Work out the finished part from the listing and answer in its coordinate system (mm). Face numbers are marked on the shaded views. A direction names the side the tool comes from. Round coordinates to 2 decimals unless told otherwise and drop trailing zeros. Order: outer loops, then holes, each group sorted by start corner. A loop starts at its lowest first (then second) coordinate and runs counter-clockwise, first axis right, second up. Notation, with made-up numbers: (29.5, 18.5) - (73.5, 18.5) arc R35 ccw to (73.5, 52.5) - close; hole circle Ø2 at (2.5, 65). An arc over 180 degrees is marked (long way). Put each result on its own line as item: value.
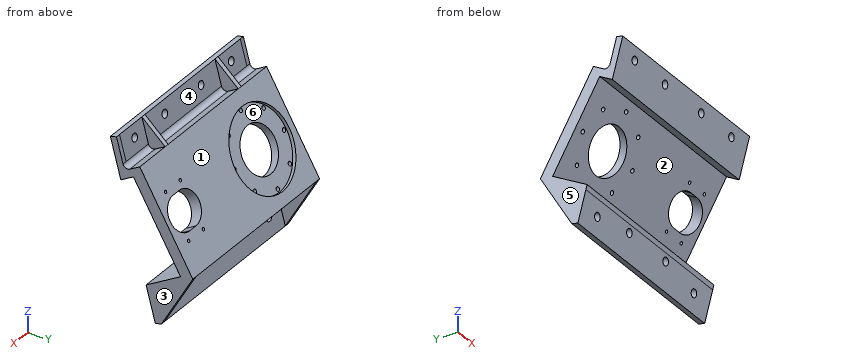
```python
from build123d import *

# Parameters (mm, degrees)
EXTRUDE_1_DEPTH      = 30
SKETCH_2_R           = 44.45
CUT_EXTRUDE_1_DEPTH  = 4
SKETCH_3_R           = 25.5
SKETCH_3_R_2         = 2.25
CUT_EXTRUDE_2_DEPTH  = 188.619295383
CUT_EXTRUDE_3_DEPTH  = 189.215302247
SKETCH_5_R           = 1.65
CUT_EXTRUDE_4_DEPTH  = 189.215302247
EXTRUDE_START        = -30
EXTRUDE_2_DEPTH      = 30
CUT_EXTRUDE_5_DEPTH  = 198.040604952
CUT_EXTRUDE_7_DEPTH  = 233.432785983
CUT_EXTRUDE_8_DEPTH  = 233.432785983
CUT_EXTRUDE_9_DEPTH  = 233.432785983
FILLET_1_R           = 5
CUT_EXTRUDE_10_DEPTH = 233.432785983
EXTRUDE_START_2      = -5
EXTRUDE_3_DEPTH      = 5
EXTRUDE_4_DEPTH      = 5
SKETCH_14_R          = 4.25
CUT_EXTRUDE_11_DEPTH = 189.364728478
SKETCH_16_W          = 43
SKETCH_16_H          = 30
CUT_EXTRUDE_12_DEPTH = 233.432785983
EXTRUDE_7_REACH      = 188.592
SKETCH_18_W          = 210
SKETCH_18_H          = 5
EXTRUDE_8_DEPTH      = 210
EXTRUDE_9_DEPTH      = 5
EXTRUDE_10_DEPTH     = 5
SKETCH_22_R          = 4.25
CUT_EXTRUDE_13_DEPTH = 187.984035343
FILLET_2_R           = 5
EXTRUDE_11_DEPTH     = 2.5
CUT_EXTRUDE_START    = -5
CUT_EXTRUDE_16_DEPTH = 5
EXTRUDE_12_DEPTH     = 2.5
CUT_EXTRUDE_18_DEPTH = 5
CUT_EXTRUDE_19_DEPTH = 366.180703078


with BuildPart() as part:
    # 草图1 → 凸台-拉伸1 (new body)
    with BuildSketch(Plane(origin=(0, 0, 0), x_dir=(1, 0, 0), z_dir=(0, 1, 0))):
        with BuildLine():
            Line((170, 31.93), (170, -31.93))
            ThreePointArc((170, -31.93), (167.781993847, -38.210172909), (162.111885646, -41.704453387))
            Line((162.111885646, -41.704453387), (15.839142344, -73.308400404))
            ThreePointArc((15.839142344, -73.308400404), (-75, 0), (15.839142344, 73.308400404))
            Line((15.839142344, 73.308400404), (162.111885646, 41.704453387))
            ThreePointArc((162.111885646, 41.704453387), (167.781993847, 38.210172909), (170, 31.93))
        make_face()
    extrude(amount=EXTRUDE_1_DEPTH)

    # 草图2 → 切除-拉伸1 (cut)
    with BuildSketch(Plane(origin=(0, 30, 0), x_dir=(1, 0, 0), z_dir=(0, 1, 0))):
        with Locations(Location((0, 0, 0), (0, 0, 270))):
            Circle(SKETCH_2_R)
    extrude(amount=-CUT_EXTRUDE_1_DEPTH, mode=Mode.SUBTRACT)

    # 草图3 → 切除-拉伸2 (cut, through all)
    with BuildSketch(Plane(origin=(0, 26, 0), x_dir=(1, 0, 0), z_dir=(0, 1, 0))):
        with Locations(Location((0, 0, 0), (0, 0, 270))):
            Circle(SKETCH_3_R)
        with Locations(Location((0, 41, 0), (0, 0, 270))):
            Circle(SKETCH_3_R_2)
        with Locations(Location((28.991378029, 28.991378029, 0), (0, 0, 270))):
            Circle(SKETCH_3_R_2)
        with Locations(Location((41, 0, 0), (0, 0, 270))):
            Circle(SKETCH_3_R_2)
        with Locations(Location((28.991378029, -28.991378029, 0), (0, 0, 270))):
            Circle(SKETCH_3_R_2)
        with Locations(Location((0, -41, 0), (0, 0, 270))):
            Circle(SKETCH_3_R_2)
        with Locations(Location((-28.991378029, -28.991378029, 0), (0, 0, 270))):
            Circle(SKETCH_3_R_2)
        with Locations(Location((-41, 0, 0), (0, 0, 270))):
            Circle(SKETCH_3_R_2)
        with Locations(Location((-28.991378029, 28.991378029, 0), (0, 0, 270))):
            Circle(SKETCH_3_R_2)
    extrude(amount=-CUT_EXTRUDE_2_DEPTH, mode=Mode.SUBTRACT)

    # 草图4 → 切除-拉伸3 (cut, through all)
    with BuildSketch(Plane(origin=(0, 30, 0), x_dir=(1, 0, 0), z_dir=(0, 1, 0))):
        with BuildLine():
            Line((124, 18.5), (134, 18.5))
            ThreePointArc((134, 18.5), (152.5, 0), (134, -18.5))
            Line((134, -18.5), (124, -18.5))
            ThreePointArc((124, -18.5), (105.5, 0), (124, 18.5))
        make_face()
    extrude(amount=-CUT_EXTRUDE_3_DEPTH, mode=Mode.SUBTRACT)

    # 草图5 → 切除-拉伸4 (cut, through all)
    with BuildSketch(Plane(origin=(0, 30, 0), x_dir=(1, 0, 0), z_dir=(0, 1, 0))):
        with Locations(Location((116.75, 25.5, 0), (0, 0, 270))):
            Circle(SKETCH_5_R)
        with Locations(Location((141.25, 25.5, 0), (0, 0, 270))):
            Circle(SKETCH_5_R)
        with Locations(Location((141.25, -25.5, 0), (0, 0, 270))):
            Circle(SKETCH_5_R)
        with Locations(Location((116.75, -25.5, 0), (0, 0, 270))):
            Circle(SKETCH_5_R)
    extrude(amount=-CUT_EXTRUDE_4_DEPTH, mode=Mode.SUBTRACT)

    # 草图6 → 凸台-拉伸2 (add)
    with BuildSketch(Plane(origin=(0, 30, 0), x_dir=(1, 0, 0), z_dir=(0, 1, 0)).offset(EXTRUDE_START)):
        with BuildLine():
            Line((158, 95), (-52, 95))
            Line((-52, 95), (-52, 54.046276467))
            ThreePointArc((-52, 54.046276467), (-20.48558667, 72.148047366), (15.839142344, 73.308400404))
            Line((15.839142344, 73.308400404), (158, 42.592874655))
            Line((158, 42.592874655), (158, 95))
        make_face()
        with BuildLine():
            ThreePointArc((15.839142344, -73.308400404), (-20.48558667, -72.148047366), (-52, -54.046276467))
            Line((-52, -54.046276467), (-52, -95))
            Line((-52, -95), (158, -95))
            Line((158, -95), (158, -42.592874655))
            Line((158, -42.592874655), (15.839142344, -73.308400404))
        make_face()
    extrude(amount=EXTRUDE_2_DEPTH)

    # 草图7 → 切除-拉伸5 (cut, through all)
    with BuildSketch(Plane(origin=(0, 30, 0), x_dir=(1, 0, 0), z_dir=(0, 1, 0))):
        with BuildLine():
            Line((-52, 54.046276467), (-52, -54.046276467))
            ThreePointArc((-52, -54.046276467), (-75, 0), (-52, 54.046276467))
        make_face()
        with BuildLine():
            Line((158, 42.592874655), (158, -42.592874655))
            Line((158, -42.592874655), (162.111885646, -41.704453387))
            ThreePointArc((162.111885646, -41.704453387), (167.781993847, -38.210172909), (170, -31.93))
            Line((170, -31.93), (170, 31.93))
            ThreePointArc((170, 31.93), (167.781993847, 38.210172909), (162.111885646, 41.704453387))
            Line((162.111885646, 41.704453387), (158, 42.592874655))
        make_face()
    extrude(amount=-CUT_EXTRUDE_5_DEPTH, mode=Mode.SUBTRACT)

    # 草图9 → 切除-拉伸7 (cut, through all)
    with BuildSketch(Plane.ZY.offset(52)):
        Polygon((-95, 20), (-60, 10.621778265), (-60, 30), (-95, 30), align=None)
    extrude(amount=-CUT_EXTRUDE_7_DEPTH, mode=Mode.SUBTRACT)

    # 草图10 → 切除-拉伸8 (cut, through all)
    with BuildSketch(Plane.ZY.offset(52)):
        Polygon((-95, 12.753066737), (-52, 1.231251463), (-52, 0), (-95, 0), align=None)
    extrude(amount=-CUT_EXTRUDE_8_DEPTH, mode=Mode.SUBTRACT)

    # 草图8 → 切除-拉伸9 (cut, through all)
    with BuildSketch(Plane.ZY.offset(52)):
        Polygon((0, 0), (52, 0), (52, 17.3), (-52, 17.3), (-52, 0), align=None)
    extrude(amount=-CUT_EXTRUDE_9_DEPTH, mode=Mode.SUBTRACT)

    # 圆角1
    fillet_1_edges = [part.edges().sort_by_distance(p)[0] for p in [
        (53, 10.621778265, -60),
    ]]
    fillet(fillet_1_edges, radius=FILLET_1_R)

    # 草图11 → 切除-拉伸10 (cut, through all)
    with BuildSketch(Plane.ZY.offset(52)):
        Polygon((-95, 12.753066737), (-93.188266684, 19.514547521), (-95, 20), align=None)
    extrude(amount=-CUT_EXTRUDE_10_DEPTH, mode=Mode.SUBTRACT)

    # 草图12 → 凸台-拉伸3 (add)
    with BuildSketch(Plane.ZY.offset(52).offset(EXTRUDE_START_2)):
        with BuildLine():
            Line((-93.188266684, 19.514547521), (-60, 30))
            Line((-60, 30), (-60, 17.137905129))
            ThreePointArc((-60, 17.137905129), (-61.956192855, 13.171138428), (-66.294095226, 12.308275998))
            Line((-66.294095226, 12.308275998), (-93.188266684, 19.514547521))
        make_face()
    extrude(amount=EXTRUDE_3_DEPTH)

    # 草图13 → 凸台-拉伸4 (add)
    with BuildSketch(Plane(origin=(158, 0, 0), x_dir=(0, 0, -1), z_dir=(1, 0, 0))):
        with BuildLine():
            Line((66.294095226, 12.308275998), (93.188266684, 19.514547521))
            Line((93.188266684, 19.514547521), (60, 30))
            Line((60, 30), (60, 17.137905129))
            ThreePointArc((60, 17.137905129), (61.956192855, 13.171138428), (66.294095226, 12.308275998))
        make_face()
    extrude(amount=-EXTRUDE_4_DEPTH)

    # 草图14 → 切除-拉伸11 (cut, through all)
    with BuildSketch(Plane(origin=(0, -5.089745962, -1.36379332), x_dir=(1, 0, 0), z_dir=(0, 0.9659258262890681, 0.2588190451025214))):
        with Locations(Location((-27, 82.063690052, 0), (0, 0, 270))):
            Circle(SKETCH_14_R)
        with Locations(Location((23, 82.063690052, 0), (0, 0, 270))):
            Circle(SKETCH_14_R)
        with Locations(Location((83, 82.063690052, 0), (0, 0, 270))):
            Circle(SKETCH_14_R)
        with Locations(Location((133, 82.063690052, 0), (0, 0, 270))):
            Circle(SKETCH_14_R)
    extrude(amount=-CUT_EXTRUDE_11_DEPTH, mode=Mode.SUBTRACT)

    # 草图16 → 切除-拉伸12 (cut, through all)
    with BuildSketch(Plane.ZY.offset(52)):
        with Locations((73.5, 15)):
            Rectangle(SKETCH_16_W, SKETCH_16_H)
    extrude(amount=-CUT_EXTRUDE_12_DEPTH, mode=Mode.SUBTRACT)

    # 凸台-拉伸7: up to this plane
    extrude_7_end = Plane(origin=(0, -11.851226746, -3.175526636), z_dir=(0, -0.9659258262890681, -0.25881904510252146))
    # 草图18 → 凸台-拉伸7 (add, up to the surface)
    with BuildSketch(Plane(origin=(0, 30, 0), x_dir=(1, 0, 0), z_dir=(0, 1, 0)), mode=Mode.PRIVATE) as extrude_7_sk1:
        with Locations((53, -54.5)):
            Rectangle(SKETCH_18_W, SKETCH_18_H)
    extrude_7_tool1 = split(extrude(extrude_7_sk1.sketch, amount=-EXTRUDE_7_REACH, mode=Mode.PRIVATE), bisect_by=extrude_7_end, keep=Keep.BOTH, mode=Mode.PRIVATE)
    add(extrude_7_tool1.solids().sort_by_distance((53, 30, 54.5))[0])

    # 草图19 → 凸台-拉伸8 (add)
    with BuildSketch(Plane.ZY.offset(52)):
        Polygon((57, -27.975210512), (90.188266684, -36.867979769), (92, -30.106498985), (57, -20.72827725), align=None)
    extrude(amount=-EXTRUDE_8_DEPTH)

    # 草图20 → 凸台-拉伸9 (add)
    with BuildSketch(Plane.ZY.offset(52)):
        Polygon((92, -30.106498985), (57, -20.72827725), (57, 30), align=None)
    extrude(amount=-EXTRUDE_9_DEPTH)

    # 草图21 → 凸台-拉伸10 (add)
    with BuildSketch(Plane(origin=(158, 0, 0), x_dir=(0, 0, -1), z_dir=(1, 0, 0))):
        Polygon((-57, 30), (-92, -30.106498985), (-57, -20.72827725), align=None)
    extrude(amount=-EXTRUDE_10_DEPTH)

    # 草图22 → 切除-拉伸13 (cut, through all)
    with BuildSketch(Plane(origin=(0, -5.089745962, -1.36379332), x_dir=(1, 0, 0), z_dir=(0, 0.9659258262890686, 0.25881904510251946))):
        with Locations(Location((-27, -77.936309948, 0), (0, 0, 270))):
            Circle(SKETCH_22_R)
        with Locations(Location((23, -69.936309948, 0), (0, 0, 270))):
            Circle(SKETCH_22_R)
        with Locations(Location((83, -69.936309948, 0), (0, 0, 270))):
            Circle(SKETCH_22_R)
        with Locations(Location((133, -77.936309948, 0), (0, 0, 270))):
            Circle(SKETCH_22_R)
    extrude(amount=-CUT_EXTRUDE_13_DEPTH, mode=Mode.SUBTRACT)

    # 圆角2
    fillet_2_edges = [part.edges().sort_by_distance(p)[0] for p in [
        (53, -20.72827725, 57),
    ]]
    fillet(fillet_2_edges, radius=FILLET_2_R)

    # 草图27 → 凸台-拉伸11 (add, symmetric)
    with BuildSketch(Plane(origin=(113.5, 0, 0), x_dir=(0, 0, -1), z_dir=(1, 0, 0))):
        with BuildLine():
            Line((60, 30), (60, 17.137905129))
            ThreePointArc((60, 17.137905129), (61.956192855, 13.171138428), (66.294095226, 12.308275998))
            Line((66.294095226, 12.308275998), (93.188266684, 19.514547521))
            Line((93.188266684, 19.514547521), (60, 30))
        make_face()
    extrude(amount=EXTRUDE_11_DEPTH, both=True)

    # 草图29 → 切除-拉伸16 (cut)
    with BuildSketch(Plane.ZY.offset(-153).offset(CUT_EXTRUDE_START)):
        with BuildLine():
            Line((-60, 17.137905129), (-60, 30))
            Line((-60, 30), (-93.188266684, 19.514547521))
            Line((-93.188266684, 19.514547521), (-66.294095226, 12.308275998))
            ThreePointArc((-66.294095226, 12.308275998), (-61.956192855, 13.171138428), (-60, 17.137905129))
        make_face()
    extrude(amount=CUT_EXTRUDE_16_DEPTH, mode=Mode.SUBTRACT)

    # 草图30 → 凸台-拉伸12 (add, symmetric)
    with BuildSketch(Plane.ZY.offset(7.5)):
        with BuildLine():
            Line((-93.188266684, 19.514547521), (-66.294095226, 12.308275998))
            ThreePointArc((-66.294095226, 12.308275998), (-61.956192855, 13.171138428), (-60, 17.137905129))
            Line((-60, 17.137905129), (-60, 30))
            Line((-60, 30), (-93.188266684, 19.514547521))
        make_face()
    extrude(amount=EXTRUDE_12_DEPTH, both=True)

    # 草图31 → 切除-拉伸18 (cut)
    with BuildSketch(Plane(origin=(-47, 0, 0), x_dir=(0, 0, -1), z_dir=(1, 0, 0))):
        with BuildLine():
            Line((66.294095226, 12.308275998), (93.188266684, 19.514547521))
            Line((93.188266684, 19.514547521), (60, 30))
            Line((60, 30), (60, 17.137905129))
            ThreePointArc((60, 17.137905129), (61.956192855, 13.171138428), (66.294095226, 12.308275998))
        make_face()
    extrude(amount=-CUT_EXTRUDE_18_DEPTH, mode=Mode.SUBTRACT)

    # 镜向2: part across plane


with BuildPart() as part_1:
    add(part.part)
    add(part.part.mirror(Plane(origin=(158, 12.753066737, -95), x_dir=(1, 0, 0), z_dir=(0, -0.2588190451025203, 0.9659258262890684))))

    # 草图32 → 切除-拉伸19 (cut, through all)
    with BuildSketch(Plane.ZY.offset(52)):
        Polygon((-93.188266684, 19.514547521), (-80.506197372, 66.84467454), (104.682069312, 17.223628034), (90.188266684, -36.867979769), (-95, 12.753066737), align=None)
    extrude(amount=-CUT_EXTRUDE_19_DEPTH, mode=Mode.SUBTRACT)


solid = part_1.part
```
1) For the marked faces 1 and 2, determine the directions among +Z, -Z, +X, -X, +Y, -Y from which every point of the face is accessible in a straight line to the end or side of a thin tool.
Findings below:
face 1: +Z, +X, -X, +Y
face 2: +X, -X
2) Straight lines are drawn through the part: L1, parallel to Y at x = 4, z = -207.5; L2, parallel to Z at x = 135, y = 81.5; L3, parallel to Y at x = 16, z = -135.5 (3 decimals). For each, find the intervals that lie inside material, in ascending order. Write a range as from..to.
Findings below:
L1: y = 82.96..93, 96.44..97.62
L2: z = -230.82..-225.05, -204.98..-186.34
L3: y = 23.605..28.605, 41.386..51.432
3) A cutting plane is placed at A-A on x = 55. Write down the section's boundary in (y, z).
Findings below:
outline: (12.75, -95) - (24.27, -138) - (38.19, -129.97) - (90.19, -220.03) - (52.14, -242) - (62.37, -280.19) - (69.14, -278.38) - (60.75, -247.08) arc R5 cw to (63.08, -241.46) - (103.69, -218.01) - (45.19, -116.69) - (34.05, -123.12) arc R5 cw to (26.72, -120.08) - (19.51, -93.19) - close
4) A cutting plane is placed at C-C on z = -236. Write down the section's boundary in (x, y), then the cut area to 3 significant figures.
Findings below:
outline: (-52, 62.53) - (158, 62.53) - (158, 93.39) - (153, 93.39) - (153, 72.53) - (-47, 72.53) - (-47, 93.39) - (-52, 93.39) - close
area: 2,310 mm2
5) For a pull along X with two mould halves and no side action, classify the marked faces 3, 4, 5 and 6 as pulls with the +X half, pulls with the -X half, needs draft (parallel to the pull), parting line crosses it, or undercut.
Findings below:
face 3: pulls with the +X half
face 4: undercut
face 5: pulls with the -X half
face 6: undercut
6) A cutting plane is placed at B-B on x = 13.5. Write down the section's boundary in (y, z), then the cut area to 3 significant figures.
Findings below:
outline: (12.75, -95) - (24.27, -138) - (38.19, -129.97) - (53.37, -156.26) - (60.91, -151.91) - (50.55, -133.97) - (54.01, -131.97) - (45.19, -116.69) - (34.05, -123.12) arc R5 cw to (26.72, -120.08) - (19.51, -93.19) - close; (52.14, -242) - (62.37, -280.19) - (69.14, -278.38) - (60.75, -247.08) arc R5 cw to (63.08, -241.46) - (103.69, -218.01) - (96.36, -205.33) - (92.9, -207.33) - (82.54, -189.38) - (75.01, -193.73) - (90.19, -220.03) - close
area: 1,620 mm2
7) Given pin 1 Ø1 at (x, z) = (103, -178) entering from -Y; pin 2 Ø1 at (x, z) = (-26.5, -126.5) entering from +Y; pin 3 Ø7.5 at (y, z) = (33, -106) entering from +X, each flat-ended and moving along its own axis, determine where each tip first touches the part or whether it passes through.
Findings below:
pin 1: stops at y = 65.63
pin 2: stops at y = 51.14
pin 3: stops at x = 116
